Study the drawing (mm; zero at the part's minimum x, y, z) and answer. A direction names the side the tool comes from. Give positions to 0.01 mm unless a question says otherwise; leave off trailing zeros. Order: outer loops, then holes, each group sorted by start corner. A loop starts at its lowest first (then second) coordinate and runs counter-clockwise, first axis right, second up. Notation, with made-up numbers: (-23.75, -9.5) - (17.25, -9.5) arc R15 ccw to (17.25, 17.5) - close; hole circle Ø9 at (53, -2.75). An arc over 180 degrees is marked (long way). Write each question's results on one line, items separated by ' | '. Start each with the question number.
1. Section B-B (x = 12.7) is taken. Give the vertices of the cut face in (y, z), and give its area (3 significant figures).
2. Section A-A (y = 18) is taken. Give the vertices of the cut face in (x, z).
3. Section D-D (x = 76) is taken. Give the vertices of the cut face in (y, z).
4. Flat-ended cylindrical pins translate along their axes: pin 1 (20.5 mm diameter, centred on x = 12.7, z = 38.1, fed in from +Y); pin 2 (6 mm diameter, centred on y = 29, z = 45.5, fed in from -X); pin 3 (5 mm diameter, centred on x = 49, y = 43, fed in from +Z). Find the tip coordinate at first contact, or state that the pin passes through.
5. Section C-C (z = 40.5) is taken. Give the vertices of the cut face in (x, y), and give its area (3 significant figures).
6. Which of the six approach directions +Z, -Z, +X, -X, +Y, -Y give full straight-line access (tool end or side, diameter ignored) to the marked faces 1 and 2?
7. Determine the mould class of the marked faces 3, 4 and 5 for opening direction Z: released by +Z, released by -Z, zero draft, split by the parting line, or undercut.
8. Find the intervals of material crossed by L1, parallel to X at y = 16, z = 38; L2, parallel to Z at x = 88.9, y = 9.5; L3, parallel to X at y = 3, z = 39.5, in increasing order.
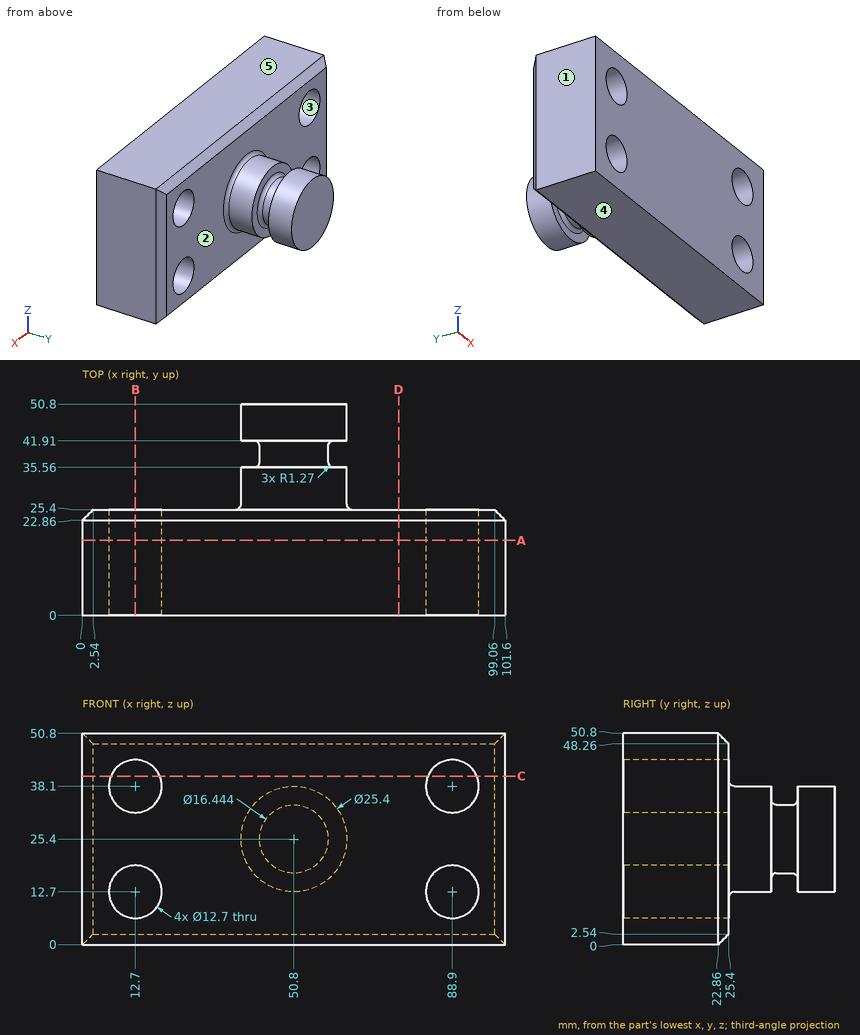
Reported:
1) outline: (0, 0) - (22.86, 0) - (25.4, 2.54) - (25.4, 6.35) - (0, 6.35) - close; (0, 19.05) - (25.4, 19.05) - (25.4, 31.75) - (0, 31.75) - close; (0, 44.45) - (25.4, 44.45) - (25.4, 48.26) - (22.86, 50.8) - (0, 50.8) - close | area: 639 mm²
2) outline: (0, 0) - (101.6, 0) - (101.6, 50.8) - (0, 50.8) - close; hole circle Ø12.7 at (12.7, 12.7); hole circle Ø12.7 at (12.7, 38.1); hole circle Ø12.7 at (88.9, 12.7); hole circle Ø12.7 at (88.9, 38.1)
3) outline: (0, 0) - (22.86, 0) - (25.4, 2.54) - (25.4, 48.26) - (22.86, 50.8) - (0, 50.8) - close
4) pin 1: y = 25.4 | pin 2: through | pin 3: z = 38.1
5) outline: (0, 0) - (6.82, 0) - (6.82, 25.4) - (2.54, 25.4) - (0, 22.86) - close; (18.58, 0) - (83.02, 0) - (83.02, 25.4) - (18.58, 25.4) - close; (94.78, 0) - (101.6, 0) - (101.6, 22.86) - (99.06, 25.4) - (94.78, 25.4) - close | area: 1,980 mm²
6) face 1: +Z, -Z, -X, +Y, -Y | face 2: +Y
7) face 3: undercut | face 4: released by -Z | face 5: released by +Z
8) L1: 0 to 6.35, 19.05 to 82.55, 95.25 to 101.6 | L2: 0 to 6.35, 19.05 to 31.75, 44.45 to 50.8 | L3: 0 to 6.51, 18.89 to 82.71, 95.09 to 101.6
